Check sheet for the drawn part. Datum: minimum x, y, z corner. Units: mm. A direction names the side the tool comes from. Round coordinates to 2 decimals unless told otherwise and drop trailing zeros. Order: outer loops, then holes, each group sorted by start corner. A loop starts at its lowest first (then second) coordinate and runs counter-clockwise, first axis right, second up. Notation, with made-up numbers: (16.25, -3) -> (45.25, -3) arc R13 ccw to (45.25, 1) -> close; hole circle Ø4 at (72.5, 72.25). An arc over 180 degrees is marked (long way). Answer as a JSON object with one key per item and string values. Group by question number.
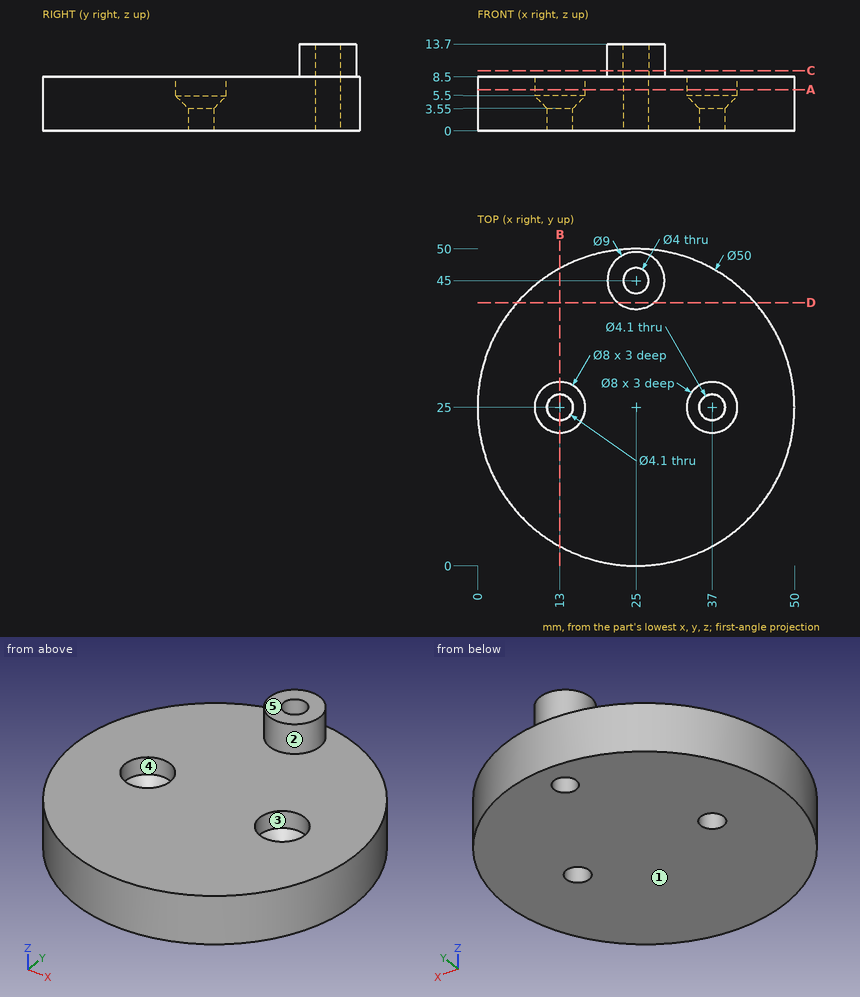
Item 1: Mould release check, pull along X, two halves, no side actions. Record for the marked faces 1, 2 and 3: pulls with the +X half, pulls with the -X half, needs draft (parallel to the pull), parting line crosses it, or undercut.
Item 2: Sectioned sample at B-B, the plane x = 13. Enter the section's corners in (y, z), then the cut area to 3 significant figures.
Item 3: Sectioned sample at C-C, the plane z = 9.5. Enter the section's corners in (x, y).
Item 4: Thickness scan on L1, parallel to X at y = 45, z = 8.75; L2, parallel to Y at x = 25, z = 7; L3, parallel to Z at x = 21, y = 21. Record the ranges inside material, lowest first.
Item 5: Sectioned sample at A-A, the plane z = 6.5. Enter the section's corners in (x, y).
Item 6: Sectioned sample at D-D, the plane y = 41.5. Enter the section's corners in (x, z).
Item 7: Set-up check for the marked faces 4 and 5: record each of +Z, -Z, +X, -X, +Y, -Y from which the full face is reachable in a straight line by a thin tool's end or side.
Item 8: Depth check by flat-ended pin: pin 1 Ø10.5 at (x, y) = (37, 25) entering from +Z; pin 2 Ø3 at (x, z) = (6, 4) entering from +Y; pin 3 Ø5 at (x, z) = (36.5, 3.5) entering from +Y. Enter the tip coordinate at first touch or a pass-through.
Result:
{
 "1": {"face 1": "needs draft", "face 2": "parting line crosses it", "face 3": "undercut"},
 "2": {"outline": "(3.07, 0) -> (22.95, 0) -> (22.95, 3.55) -> (21, 5.5) -> (21, 8.5) -> (3.07, 8.5) -> close; (27.05, 0) -> (46.93, 0) -> (46.93, 8.5) -> (29, 8.5) -> (29, 5.5) -> (27.05, 3.55) -> close", "area": "322 mm2"},
 "3": {"outline": "circle Ø9 at (25, 45); hole circle Ø4 at (25, 45)"},
 "4": {"L1": "x = 20.5 to 23, 27 to 29.5", "L2": "y = 0 to 43, 47 to 50", "L3": "z = 0 to 8.5"},
 "5": {"outline": "circle Ø50 at (25, 25); hole circle Ø8 at (13, 25); hole circle Ø4 at (25, 45); hole circle Ø8 at (37, 25)"},
 "6": {"outline": "(6.22, 0) -> (43.78, 0) -> (43.78, 8.5) -> (27.83, 8.5) -> (27.83, 13.7) -> (22.17, 13.7) -> (22.17, 8.5) -> (6.22, 8.5) -> close"},
 "7": {"face 4": "+Z", "face 5": "+Z, +X, -X, +Y, -Y"},
 "8": {"pin 1": "stops at z = 8.5", "pin 2": "stops at y = 42.85", "pin 3": "stops at y = 48.32"}
}
